CAD build for the part. Positions are in the model's coordinates, mm. Face numbers are marked on the shaded views. Coordinates: 2 decimals unless noted, no trailing zeros. Write each loop counter-clockwise with the first axis right and the second up, starting at its lowest first coordinate (ties: lowest second). Pieces come first, ordered by that corner, then holes. Notation, with made-up numbers: (82, -19) - (103, -19) arc R19 ccw to (103, 7) - close; hole circle Ø7 at (27.5, 29). An arc over 180 degrees is marked (long way). Answer in a Markdown table with one row per item. Add a question column.
Q1. Band-saw the part on C-C (y = 0.8). List the corners of the cut face in (x, z).
Q2. Drill centre lines: line 1 along X through (y, z) = (1, 0); line 2 along Z through (x, y) = (-3, 0.25); line 3 along X through (y, z) = (1.4, -2.5). Where is each one in solid material? Low to high. Write a range as from..to.
Q3. Two-plate mould, pull along Z, no slides. Class the marked faces 1, 2 and 3: +Z half, -Z half, draft (parallel to the pull), parting line (faces both ways), or undercut.
Q4. Band-saw the part on D-D (y = 0.15). List the corners of the cut face in (x, z) (3 decimals), and give its area (3 significant figures).
Q5. Band-saw the part on A-A (x = 0). List the corners of the cut face in (y, z), and give its area (3 significant figures).
Q6. Band-saw the part on B-B (z = 0). List the corners of the cut face in (x, y).
```python
from build123d import *

# Parameters (mm, degrees)
SKETCH_1_R      = 3.5
EXTRUDE_1_DEPTH = 2
FILLET_1_R      = 1
CHAMFER_1_SIZE  = 0.5


with BuildPart() as part:
    # 草图1 → 凸台-拉伸1 (new body)
    with BuildSketch(Plane(origin=(0, 0, 0), x_dir=(1, 0, 0), z_dir=(0, 1, 0))):
        Polygon((5.773502692, 0), (2.886751346, 5), (-2.886751346, 5), (-5.773502692, 0), (-2.886751346, -5), (2.886751346, -5), align=None)
        with Locations(Location((0, 0, 0), (0, 0, 270))):
            Circle(SKETCH_1_R, mode=Mode.SUBTRACT)
    extrude(amount=EXTRUDE_1_DEPTH)

    # 圆角1
    fillet_1_edges = [part.edges().sort_by_distance(p)[0] for p in [
        (2.886751346, 1, 5),
        (-2.886751346, 1, 5),
        (-5.773502692, 1, 0),
        (-2.886751346, 1, -5),
        (2.886751346, 1, -5),
        (5.773502692, 1, 0),
    ]]
    fillet(fillet_1_edges, radius=FILLET_1_R)

    # 倒角1
    chamfer_1_edges = [part.edges().sort_by_distance(p)[0] for p in [
        (0, 0, -3.5),
        (0, 2, -3.5),
        (-4.330127019, 0, 2.5),
        (-4.330127019, 2, 2.5),
        (4.330127019, 0, 2.5),
        (0, 0, 5),
        (-4.330127019, 0, -2.5),
        (0, 0, -5),
        (4.330127019, 0, -2.5),
        (-2.809401077, 0, 4.866025404),
        (2.809401077, 0, 4.866025404),
        (5.618802154, 0, 0),
        (2.809401077, 0, -4.866025404),
        (-2.809401077, 0, -4.866025404),
        (-5.618802154, 0, 0),
        (-4.330127019, 2, -2.5),
        (4.330127019, 2, 2.5),
        (4.330127019, 2, -2.5),
        (0, 2, -5),
        (0, 2, 5),
        (-2.809401077, 2, 4.866025404),
        (2.809401077, 2, 4.866025404),
        (5.618802154, 2, 0),
        (2.809401077, 2, -4.866025404),
        (-2.809401077, 2, -4.866025404),
        (-5.618802154, 2, 0),
    ]]
    chamfer(chamfer_1_edges, length=CHAMFER_1_SIZE)


solid = part.part
```
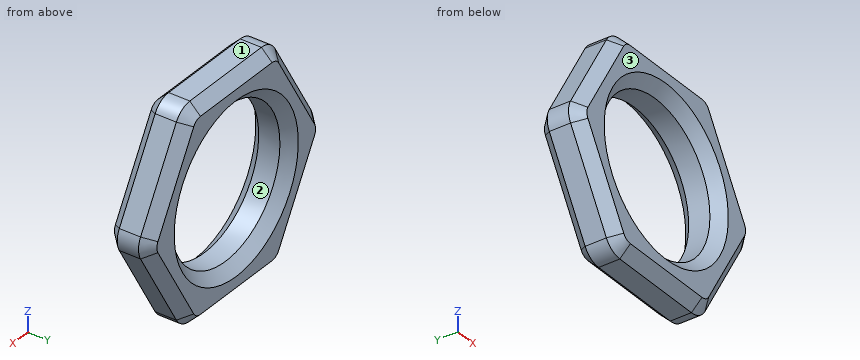
Checked values:
| question | item | result |
|---|---|---|
| 1 | outline | (-5.48, -0.5) - (-3.18, -4.5) arc R1 ccw to (-2.31, -5) - (2.31, -5) arc R1 ccw to (3.18, -4.5) - (5.48, -0.5) arc R1 ccw to (5.48, 0.5) - (3.18, 4.5) arc R1 ccw to (2.31, 5) - (-2.31, 5) arc R1 ccw to (-3.18, 4.5) - (-5.48, 0.5) arc R1 ccw to start; hole circle Ø7 at (0, 0) |
| 2 | line 1 | x = -5.62..-3.5, 3.5..5.62 |
| 2 | line 2 | z = -4.3..-2.25, 2.25..4.3 |
| 2 | line 3 | x = -4.33..-2.45, 2.45..4.33 |
| 3 | face 1 | +Z half |
| 3 | face 2 | undercut |
| 3 | face 3 | draft |
| 4 | outline | (-5.182, -0.325) - (-2.872, -4.325) arc R0.65 ccw to (-2.309, -4.65) - (2.309, -4.65) arc R0.65 ccw to (2.872, -4.325) - (5.182, -0.325) arc R0.65 ccw to (5.182, 0.325) - (2.872, 4.325) arc R0.65 ccw to (2.309, 4.65) - (-2.309, 4.65) arc R0.65 ccw to (-2.872, 4.325) - (-5.182, 0.325) arc R0.65 ccw to start; hole circle Ø7.7 at (0, 0) |
| 4 | area | 28.2 mm² |
| 5 | outline | (0, -4.5) - (0.5, -5) - (1.5, -5) - (2, -4.5) - (2, -4) - (1.5, -3.5) - (0.5, -3.5) - (0, -4) - close; (0, 4) - (0.5, 3.5) - (1.5, 3.5) - (2, 4) - (2, 4.5) - (1.5, 5) - (0.5, 5) - (0, 4.5) - close |
| 5 | area | 5.00 mm² |
| 6 | outline | (-5.62, 0.5) - (-5.12, 0) - (-4, 0) - (-3.5, 0.5) - (-3.5, 1.5) - (-4, 2) - (-5.12, 2) - (-5.62, 1.5) - close; (3.5, 0.5) - (4, 0) - (5.12, 0) - (5.62, 0.5) - (5.62, 1.5) - (5.12, 2) - (4, 2) - (3.5, 1.5) - close |
